Autodesk Inventor part; units mm, degrees
ref_plane "YZ Plane" through (0, 0, 0) normal (1, 0, 0) x (0, 1, 0)
ref_plane "XZ Plane" through (0, 0, 0) normal (0, 1, 0) x (-1, 0, 0)
ref_plane "XY Plane" through (0, 0, 0) normal (0, 0, 1) x (1, 0, 0)
sketch "Sketch1" plane through (0, 0, 0) normal (0, 1, 0) x (-1, 0, 0)
  circle A0 centre (0, 0) radius 6.35
  dimension "d0" = 12.7
extrude "Extrusion1" add sketch "Sketch1" along normal blind 38.1
sketch "Sketch2" plane through (0, 38.1, 0) normal (0, 1, 0) x (1, 0, 0)
  circle A0 centre (0, 0) radius 7.112
  dimension "d3" = 14.224
extrude "Extrusion2" add sketch "Sketch2" along normal blind 2.54
sketch "Sketch3" plane through (0, 0, 0) normal (0, -1, 0) x (1, 0, 0)
  line L0 (-6.35, -2.794) -> (6.35, -2.794)
  line L1 (6.35, -2.794) -> (6.35, 2.794)
  line L2 (6.35, 2.794) -> (-6.35, 2.794)
  line L3 (-6.35, 2.794) -> (-6.35, -2.794)
  point P0 (0, 0)
  dimension "d6" = 5.588
extrude "Extrusion3" cut sketch "Sketch3" against normal blind 1.27
sketch "Sketch4" plane through (0, 1.27, 0) normal (0, -1, 0) x (1, 0, 0)
  line L0 (5.7023, -2.794) -> (-5.7023, -2.794)
  line L1 (5.7023, -2.794) -> (-11.0724, -2.794)
  line L2 (-11.0724, -2.794) -> (-11.0724, 8.6812)
  line L3 (-11.0724, 8.6812) -> (5.7023, 8.6812)
  line L4 (5.7023, 8.6812) -> (5.7023, -2.794)
  line L5 (-11.0724, -2.794) -> (15.5291, -2.794)
  line L6 (15.5291, -2.794) -> (15.5291, 8.6812)
  line L7 (15.5291, 8.6812) -> (-11.0724, 8.6812)
  line L8 (-11.0724, 8.6812) -> (-11.0724, -2.794)
  point P0 (0, 0)
sketch "Sketch5" plane through (0, 1.27, 0) normal (0, -1, 0) x (1, 0, 0)
  line L0 (8.174, 2.794) -> (-7.6116, 2.794)
  line L1 (-7.6116, 2.794) -> (-7.6116, -2.794)
  line L2 (-7.6116, -2.794) -> (8.174, -2.794)
  line L3 (8.174, -2.794) -> (8.174, 2.794)
  point P0 (0, 0)
extrude "Extrusion4" cut sketch "Sketch5" against normal blind 0.5588
extrude "Extrusion5" cut sketch "Sketch4" against normal up to next
sketch "Sketch6" plane through (0, 0, 0) normal (0, -1, 0) x (1, 0, 0)
  line L0 (14.7281, 0) -> (-10.6227, 0)
  line L1 (-10.6227, 0) -> (-10.6227, 18.3203)
  line L2 (-10.6227, 18.3203) -> (14.7281, 18.3203)
  line L3 (14.7281, 18.3203) -> (14.7281, 0)
  point P0 (0, 0)
extrude "Extrusion6" cut sketch "Sketch6" against normal blind 25.4
sketch "Sketch7" plane through (0, 0, 0) normal (0, -1, 0) x (1, 0, 0)
  arc A0 (-5.7023, -2.794) -> (5.7023, -2.794) centre (0, 0) ccw
  line L0 (-5.7023, -2.794) -> (-6.5402, -2.794)
  line L1 (5.7023, -2.794) -> (-5.7023, -2.794)
  arc A1 (-5.7023, -2.794) -> (5.7023, -2.794) centre (0, 0) ccw
extrude "Extrusion7" add sketch "Sketch7" along normal blind 7.62
properties part number "Pin Place holder"
Here's how the part is built. I have some questions about the finished solid (model axes, mm). A direction names the side the tool comes from. Give positions to 0.01 mm unless a question says otherwise; leave off trailing zeros. Loops run counter-clockwise (first coordinate to the right, second up) from the corner with the lowest first, then second, coordinate; pieces in that order, holes last. Notation, with made-up numbers: M 20.5,-18.75 L 34.5,-18.75 A23 ccw 34.5,3.25 Z; hole C -12.75,-28.75 d11. An arc over 180 degrees is marked long. Use one line per item in the form item = value. Start each with the question number.
Q1. I need wall thicknesses on line 1 along Y through (x, z) = (-1.25, -6.85); line 2 along Z through (x, y) = (0.25, 31); line 3 along X through (y, z) = (37, -3.95). Which ranges of each line are inside material? Lowest first, please.
Q2. Which directions (+Z, -Z, +X, -X, +Y, -Y) give clear straight access to the entire face, cutting with the end or side of a thin tool? Please do faces 1 (the flat face through (0, 40.64, -5)), 2 (the cylindrical face through (-0.1, 18.78, -6.35)).
Q3. If we section it at C-C (y = 18): Write out the boundary of the cut face in (x, z), then the cut area to 3 significant figures.
Q4. Will this pin go through, and if not, where does the flat tip stop? pin 1 Ø5 at (x, y) = (-5, 20.5) entering from -Z.
Taken from the geometry:
q1.line_1 = 38.1 to 40.64
q1.line_2 = -6.35 to -2.79
q1.line_3 = -4.97 to 4.97
q2.face_1 = +Z, -Z, +X, -X, +Y
q2.face_2 = -Z, -Y
q3.outline = M -5.7,-2.79 A6.35 ccw 5.7,-2.79 Z
q3.area = 29.0 mm^2
q4.pin_1 = -5.84
